```python
from build123d import *

# Parameters (mm, degrees)
ESQUISSE1_R         = 17.7
ESQUISSE1_R_2       = 12.7
BOSS_EXTRU_1_DEPTH  = 8.78
ESQUISSE2_R         = 38
ESQUISSE2_R_2       = 11.2
BOSS_EXTRU_2_DEPTH  = 47.8
CHANFREIN3_SIZE     = 11.200084029
CHANFREIN3_SIZE_2   = 49.8
SKETCH7_R           = 38
SKETCH7_R_2         = 26
CUT_EXTRUDE2_DEPTH  = 3
CIRPATTERN1_COUNT   = 4
CIRPATTERN2_COUNT   = 3
SKETCH23_R          = 13.7
SKETCH23_R_2        = 12.6
BOSS_EXTRUDE1_DEPTH = 0.3
LPATTERN1_COUNT     = 8
LPATTERN1_PITCH     = 5


with BuildPart() as part:
    # Esquisse1 → Boss.-Extru.1 (new body)
    with BuildSketch(Plane.XY):
        Circle(ESQUISSE1_R)
        Circle(ESQUISSE1_R_2, mode=Mode.SUBTRACT)
    extrude(amount=BOSS_EXTRU_1_DEPTH)

    # Esquisse2 → Boss.-Extru.2 (add)
    with BuildSketch(Plane(origin=(0, 0, 0), x_dir=(-1, 0, 0), z_dir=(0, 0, -1))):
        with Locations(Location((0, 0, 0), (0, 0, 180))):
            Circle(ESQUISSE2_R)
        with Locations(Location((0, 0, 0), (0, 0, 180))):
            Circle(ESQUISSE2_R_2, mode=Mode.SUBTRACT)
    extrude(amount=BOSS_EXTRU_2_DEPTH)

    # Chanfrein3
    # the kernel refuses this chamfer: 49.8, 11.200084029 mm, written as the material it takes off along each edge
    with BuildSketch(Plane(origin=(0, 0, -47.8), x_dir=(1, 0, 0), z_dir=(0, 1, 0))) as chanfrein3_piece_1:
        Polygon((11.2 + CHANFREIN3_SIZE, 0), (11.2, -CHANFREIN3_SIZE_2), (11.2, 0), align=None)
    revolve(axis=Axis((0, 0, -47.8), (0, 0, -1)), mode=Mode.SUBTRACT)

    # Sketch7 → Cut-Extrude2 (cut)
    with BuildSketch(Plane.XY):
        Circle(SKETCH7_R)
        Circle(SKETCH7_R_2, mode=Mode.SUBTRACT)
    cut_extrude2 = extrude(amount=-CUT_EXTRUDE2_DEPTH, mode=Mode.SUBTRACT)

    # Sketch19 → #4-40 Tapped Hole1 (revolve, cut)
    with BuildSketch(Plane(origin=(13.743816873, -26.666598917, -47.8), x_dir=(0, 1, 0), z_dir=(1, 0, 0))):
        Polygon((0, 0), (0, 5.679152758), (1.1303, 5), (1.1303, 0), align=None)
    f_4_40_tapped_hole1 = revolve(axis=Axis((13.743816873, -26.666598917, -54.15), (0, 0, 1)), mode=Mode.SUBTRACT)

    # CirPattern1: #4-40 Tapped Hole1 ×4 about axis
    cirpattern1_axis = Axis((0, 0, 0), (0, 0, 1))
    for i in range(1, CIRPATTERN1_COUNT):
        add(f_4_40_tapped_hole1.rotate(cirpattern1_axis, i * 360 / CIRPATTERN1_COUNT), mode=Mode.SUBTRACT)

    # Sketch22 → #4-40 Tapped Hole2 (revolve, cut)
    with BuildSketch(Plane(origin=(7.032252966, -13.644409779, 8.78), x_dir=(0, -1, 0), z_dir=(1, 0, 0))):
        Polygon((0, 0), (0, 5.679152758), (1.1303, 5), (1.1303, 0), align=None)
    f_4_40_tapped_hole2 = revolve(axis=Axis((7.032252966, -13.644409779, 15.13), (0, 0, -1)), mode=Mode.SUBTRACT)

    # CirPattern2: #4-40 Tapped Hole2 ×3 about axis
    cirpattern2_axis = Axis((0, 0, 0), (0, 0, 1))
    for i in range(1, CIRPATTERN2_COUNT):
        add(f_4_40_tapped_hole2.rotate(cirpattern2_axis, i * 360 / CIRPATTERN2_COUNT), mode=Mode.SUBTRACT)

    # Sketch23 → Boss-Extrude1 (add)
    with BuildSketch(Plane.XY):
        Circle(SKETCH23_R)
        Circle(SKETCH23_R_2, mode=Mode.SUBTRACT)
    extrude(amount=BOSS_EXTRUDE1_DEPTH)

    # LPattern1: Cut-Extrude2 ×8
    with Locations(*[(0, 0, -i * LPATTERN1_PITCH) for i in range(1, LPATTERN1_COUNT)]):
        add(cut_extrude2, mode=Mode.SUBTRACT)


solid = part.part
```
Can you work these out from the model? Positions are in its coordinate system, mm. A direction names the side the tool comes from. Round coordinates to 2 decimals unless told otherwise and drop trailing zeros. Loops run counter-clockwise (first coordinate to the right, second up) from the corner with the lowest first, then second, coordinate; pieces in that order, holes last. Notation, with made-up numbers: M 53,-28.75 L 68,-28.75 A19 cw 68,-10.75 Z; hole C 60,37 d8. An arc over 180 degrees is marked long. Write item = value, one per line. Start each with the question number.
(1) I'm going to push flat-ended pins straight in: P1, Ø20, axis at x = 1.5, y = -3, coming from the +Z side; P2, Ø1, axis at y = 8.5, z = -1, coming from the -X side; P3, Ø12, axis at y = 15.5, z = -15.5, coming from the +X side; P4, Ø5, axis at x = -21, z = -21, coming from the +Y side. Where does each tip first touch, or does it pass through?
(2) I need wall thicknesses on line 1 along Y through (x, z) = (0, 0.15); line 2 along X through (y, z) = (3, -31); line 3 along Y through (x, z) = (0, 5). Which ranges of each line are inside material? Lowest first, please.
(3) Which directions (+Z, -Z, +X, -X, +Y, -Y) give clear straight access to the entire face, cutting with the end or side of a thin tool? Please do faces 1 (the face through (-8.238, 37.096, -33.986)), 2 (the face through (-20.633, -15.821, -6.479)), 3 (the face through (-20.633, -15.821, -1.479)).
(4) If we mould it in two halves opening along Y, with no side actions, what happens to faces 4 (the face through (-20.633, -15.821, -11.479)), 5 (the face through (25, -8, -10)), 6 (the face through (-13.735, 26.863, -42.239))? For each: released by +Y, released by -Y, zero draft, split by the parting line, or undercut.
(5) Suppose I cut it at B-B on z = -16.5. Write out the boundary of the cut face in (x, y).
(6) Suppose I cut it at A-A on x = -31. Give the number of separate pieces and of enclosed holes in the cut face, plus the area to 3 significant figures.
Answer block:
q1.P1 = 8.78
q1.P2 = -24.74
q1.P3 = 36.79
q1.P4 = 33.08
q2.line_1 = -17.7 to -12.6, 12.6 to 17.7
q2.line_2 = -25.83 to -18.38, 18.38 to 25.83
q2.line_3 = -17.7 to -12.7, 12.7 to 17.7
q3.face_1 = +Z, -Z
q3.face_2 = none
q3.face_3 = +Z
q4.face_4 = split by the parting line
q4.face_5 = zero draft
q4.face_6 = undercut
q5.outline = C 0,0 d52; hole C 0,0 d30.72
q6.separate_pieces = 8
q6.enclosed_holes = 0
q6.area = 1,050 mm²
